```python
from build123d import *

# Parameters (mm, degrees)
SKETCH_1_W                       = 49.5
SKETCH_1_H                       = 49.5
SKETCH_1_R                       = 23.75
EXTRUDE_1_DEPTH                  = 11.98
SKETCH_2_R                       = 3
CUT_EXTRUDE_1_DEPTH              = 2.5
SKETCH_3_R                       = 1.6
CUT_EXTRUDE_2_DEPTH              = 10.48
CUT_EXTRUDE_3_DEPTH              = 12.98
CUT_EXTRUDE_4_DEPTH              = 9.5
PATTERN_CIRCULAR_1_COUNT         = 4
SKETCH_7_R                       = 12.5
EXTRUDE_2_DEPTH                  = 2
EXTRUDE_3_DEPTH                  = 2
FILLET_2_R                       = 2
PATTERN_CIRCULAR_2_COUNT         = 3
FILLET_2_OF_PATTERN_CIRCULAR_2_R = 2
SKETCH_9_R                       = 2
EXTRUDE_4_DEPTH                  = 7
CUT_EXTRUDE_5_DEPTH              = 9.5
EXTRUDE_5_DEPTH                  = 10


with BuildPart() as part:
    # Sketch 1 → Extrude 1 (new body)
    with BuildSketch(Plane(origin=(0, 0, 0), x_dir=(1, 0, 0), z_dir=(0, 1, 0))):
        Rectangle(SKETCH_1_W, SKETCH_1_H)
        Circle(SKETCH_1_R, mode=Mode.SUBTRACT)
    extrude(amount=EXTRUDE_1_DEPTH)

    # Sketch 2 → Cut-Extrude 1 (cut)
    with BuildSketch(Plane(origin=(0, 11.98, 0), x_dir=(1, 0, 0), z_dir=(0, 1, 0))):
        with Locations((-19.798989873, 19.798989873)):
            Circle(SKETCH_2_R)
    cut_extrude_1 = extrude(amount=-CUT_EXTRUDE_1_DEPTH, mode=Mode.SUBTRACT)

    # Sketch 3 → Cut-Extrude 2 (cut, through all)
    with BuildSketch(Plane(origin=(0, 9.48, 0), x_dir=(1, 0, 0), z_dir=(0, 1, 0))):
        with Locations((-19.798989873, 19.798989873)):
            Circle(SKETCH_3_R)
    cut_extrude_2 = extrude(amount=-CUT_EXTRUDE_2_DEPTH, mode=Mode.SUBTRACT)

    # Sketch 4 → Cut-Extrude 3 (cut, through all)
    with BuildSketch(Plane(origin=(0, 11.98, 0), x_dir=(1, 0, 0), z_dir=(0, 1, 0))):
        with BuildLine():
            Line((-24.75, 19.798989873), (-24.75, 24.75))
            Line((-24.75, 24.75), (-19.798989873, 24.75))
            ThreePointArc((-19.798989873, 24.75), (-23.299882708, 23.299882708), (-24.75, 19.798989873))
        make_face()
    cut_extrude_3 = extrude(amount=-CUT_EXTRUDE_3_DEPTH, mode=Mode.SUBTRACT)

    # Sketch 5 → Cut-Extrude 4 (cut)
    with BuildSketch(Plane(origin=(0, 11.98, 0), x_dir=(1, 0, 0), z_dir=(0, 1, 0))):
        with BuildLine():
            Line((-23.75, 18.375988463), (-19.980393233, 14.606381696))
            ThreePointArc((-19.980393233, 14.606381696), (-22.196566868, 10.948740533), (-23.75, 6.964194139))
            Line((-23.75, 6.964194139), (-23.75, 18.375988463))
        make_face()
        with BuildLine():
            Line((-18.375988463, 23.75), (-6.964194139, 23.75))
            ThreePointArc((-6.964194139, 23.75), (-10.948740533, 22.196566868), (-14.606381696, 19.980393233))
            Line((-14.606381696, 19.980393233), (-18.375988463, 23.75))
        make_face()
    cut_extrude_4 = extrude(amount=-CUT_EXTRUDE_4_DEPTH, mode=Mode.SUBTRACT)

    # Pattern Circular 1: Cut-Extrude 1, Cut-Extrude 2, Cut-Extrude 3, Cut-Extrude 4 ×4 about axis
    pattern_circular_1_axis = Axis((0, 0, 0), (0, 1, 0))
    for i in range(1, PATTERN_CIRCULAR_1_COUNT):
        add(cut_extrude_1.rotate(pattern_circular_1_axis, i * 360 / PATTERN_CIRCULAR_1_COUNT), mode=Mode.SUBTRACT)
        add(cut_extrude_2.rotate(pattern_circular_1_axis, i * 360 / PATTERN_CIRCULAR_1_COUNT), mode=Mode.SUBTRACT)
        add(cut_extrude_3.rotate(pattern_circular_1_axis, i * 360 / PATTERN_CIRCULAR_1_COUNT), mode=Mode.SUBTRACT)
        add(cut_extrude_4.rotate(pattern_circular_1_axis, i * 360 / PATTERN_CIRCULAR_1_COUNT), mode=Mode.SUBTRACT)



with BuildPart() as body_2:
    # Sketch 7 → Extrude 2 (new body)
    with BuildSketch(Plane.XZ):
        Circle(SKETCH_7_R)
    extrude(amount=-EXTRUDE_2_DEPTH)


with BuildPart() as part_1:
    add(part.part)

    add(body_2.part)  # Extrude 3 merges body 2
    # Sketch 8 → Extrude 3 (add)
    with BuildSketch(Plane.XZ):
        with BuildLine():
            Line((23.68169124, -1.8), (12.369721096, -1.8))
            ThreePointArc((12.369721096, -1.8), (12.5, 0), (12.369721096, 1.8))
            Line((12.369721096, 1.8), (23.68169124, 1.8))
            ThreePointArc((23.68169124, 1.8), (23.75, 0), (23.68169124, -1.8))
        make_face()
    extrude_3 = extrude(amount=-EXTRUDE_3_DEPTH)

    # Fillet 2
    fillet_2_edges = [part_1.edges().sort_by_distance(p)[0] for p in [
        (23.68169124, 1, 1.8),
        (23.68169124, 1, -1.8),
        (12.369721096, 1, -1.8),
        (12.369721096, 1, 1.8),
    ]]
    fillet(fillet_2_edges, radius=FILLET_2_R)

    # Pattern Circular 2: Extrude 3 ×3 about axis
    pattern_circular_2_axis = Axis((0, 0, 0), (0, 1, 0))
    for i in range(1, PATTERN_CIRCULAR_2_COUNT):
        add(extrude_3.rotate(pattern_circular_2_axis, i * 360 / PATTERN_CIRCULAR_2_COUNT))

    # Fillet 2 of Pattern Circular 2
    fillet_2_of_pattern_circular_2_edges = [part_1.edges().sort_by_distance(p)[0] for p in [
        (-10.281999893, 1, -21.408946219),
        (-13.399691347, 1, -19.608946219),
        (-7.743706275, 1, -9.812492707),
        (-4.626014821, 1, -11.612492707),
        (-13.399691347, 1, 19.608946219),
        (-10.281999893, 1, 21.408946219),
        (-4.626014821, 1, 11.612492707),
        (-7.743706275, 1, 9.812492707),
    ]]
    fillet(fillet_2_of_pattern_circular_2_edges, radius=FILLET_2_OF_PATTERN_CIRCULAR_2_R)

    # Sketch 9 → Extrude 4 (add)
    with BuildSketch(Plane(origin=(0, 2, 0), x_dir=(1, 0, 0), z_dir=(0, 1, 0))):
        Circle(SKETCH_9_R)
    extrude(amount=EXTRUDE_4_DEPTH)

    # Sketch 10 → Cut-Extrude 5 (cut)
    with BuildSketch(Plane(origin=(0, 11.98, 0), x_dir=(1, 0, 0), z_dir=(0, 1, 0))):
        with BuildLine():
            Line((-14.606381696, 19.980393233), (-19.375988463, 24.75))
            Line((-19.375988463, 24.75), (0, 24.75))
            ThreePointArc((0, 24.75), (-7.68270029, 23.527401392), (-14.606381696, 19.980393233))
        make_face()
    extrude(amount=-CUT_EXTRUDE_5_DEPTH, mode=Mode.SUBTRACT)

    # Sketch 11 → Extrude 5 (add)
    with BuildSketch(Plane(origin=(0, 2.48, 0), x_dir=(1, 0, 0), z_dir=(0, 1, 0))):
        with BuildLine():
            Line((-13.662941725, 23.240819528), (-13.691818706, 23.240819528))
            ThreePointArc((-13.691818706, 23.240819528), (-14.877380215, 23.109984827), (-13.691818706, 22.979150126))
            Line((-13.691818706, 22.979150126), (-13.662941725, 22.979150126))
            ThreePointArc((-13.662941725, 22.979150126), (-12.477380215, 23.109984827), (-13.662941725, 23.240819528))
        make_face()
    extrude(amount=EXTRUDE_5_DEPTH)


solid = part_1.part
```
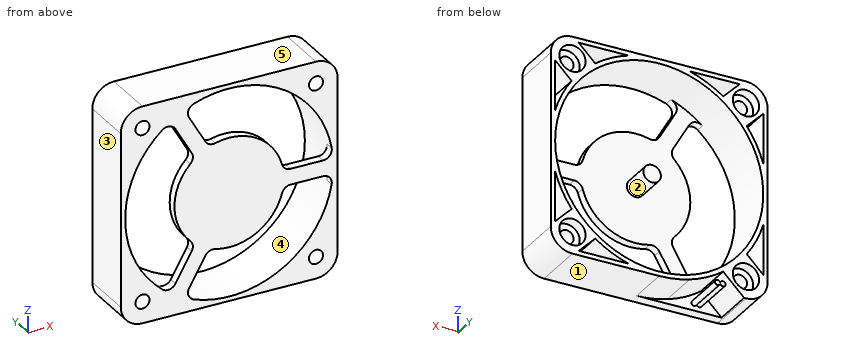
Model file for the job. Use its own axes, mm. Face numbers are marked on the shaded views. A direction names the side the tool comes from. Coordinates: 2 decimals unless noted, no trailing zeros. Loops run counter-clockwise (first coordinate to the right, second up) from the corner with the lowest first, then second, coordinate; pieces in that order, holes last. Notation, with made-up numbers: M 24.5,79.25 L 36.5,79.25 A24 ccw 36.5,107.25 Z; hole C 2.25,21.5 d2. An arc over 180 degrees is marked long. Use CSV: the item, a comma, the result in double quotes. Start each with the question number.
1. Tool access for the marked faces 1 and 2: list every direction of +Z, -Z, +X, -X, +Y, -Y with a clear straight run to the whole face (end or side of a thin tool).
2. Band-saw the part on D-D, the plane x = 22. List the corners of the cut face in (y, z), then the cut area to 3 significant figures.
3. Probe probe 1 along Z at (x, y) = (0, 7.25); probe 2 along Z at (x, y) = (21, 11); probe 3 along X at (y, z) = (1.75, 3.5). List the from-to ranges inside material, lowest first. Write a range as [from, to].
4. Flat gauge pins, fed straight in: pin 1 (6 mm diameter, centred on x = -1, z = -7.5, fed in from +Y); pin 2 (7 mm diameter, centred on x = 19.8, z = 19.8, fed in from +Y). Where does each tip first touch, or does it go through?
5. Band-saw the part on A-A, the plane z = 0. List the corners of the cut face in (x, y).
6. Band-saw the part on B-B, the plane y = 11. Give the number of separate pieces and of enclosed holes in the cut face, then the cut area to 3 significant figures.
7. Two-plate mould, pull along Z, no slides. Class the marked faces 3, 4 and 5: pulls with the +Z half, pulls with the -Z half, needs draft (parallel to the pull), parting line crosses it, or undercut.
Entries:
1,face 1,"-Z, +X, -X, +Y, -Y"
1,face 2,"+Y"
2,outline,"M 0,-24.23 L 11.98,-24.23 L 11.98,-21.84 L 9.48,-21.84 L 9.48,-17.76 L 11.98,-17.76 L 11.98,-16.63 L 2.48,-16.63 L 2.48,-11.34 L 11.98,-11.34 L 11.98,-8.95 L 0,-8.95 Z; M 0,-1.89 L 2,-1.89 L 2,1.89 L 0,1.89 Z; M 0,8.95 L 11.98,8.95 L 11.98,11.34 L 2.48,11.34 L 2.48,16.63 L 11.98,16.63 L 11.98,17.76 L 9.48,17.76 L 9.48,21.84 L 11.98,21.84 L 11.98,24.23 L 0,24.23 Z"
2,area,"253 mm2"
3,probe 1,"z = [-24.75, -23.75], [-2, 2], [23.75, 24.75]"
3,probe 2,"z = [-24.6, -22.55], [-17.05, -15.63], [-13.1, -11.09], [11.09, 13.1], [15.63, 17.05], [22.55, 24.6]"
3,probe 3,"x = [-24.75, -23.49], [-12, 12], [23.39, 24.75]"
4,pin 1,"stops at y = 2"
4,pin 2,"stops at y = 11.98"
5,outline,"M -24.75,0 L -23.75,0 L -23.75,11.98 L -24.75,11.98 Z; M -12.5,0 L 24.75,0 L 24.75,11.98 L 23.75,11.98 L 23.75,2 L 2,2 L 2,9 L -2,9 L -2,2 L -12.5,2 Z"
6,separate pieces,"2"
6,enclosed holes,"12"
6,area,"377 mm2"
7,face 3,"needs draft"
7,face 4,"undercut"
7,face 5,"pulls with the +Z half"
